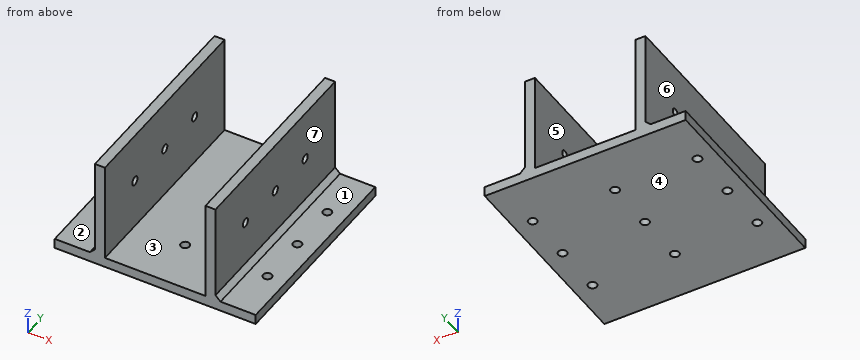
```python
from build123d import *

# Parameters (mm, degrees)
SKETCH1_W               = 100
SKETCH1_H               = 100
BOSS_EXTRUDE1_DEPTH     = 5
SKETCH2_W               = 5
SKETCH2_H               = 100
BOSS_EXTRUDE2_DEPTH     = 50
SKETCH3_R               = 2.15
CUT_EXTRUDE1_DEPTH      = 10
LPATTERN1_COUNT         = 3
LPATTERN1_PITCH         = 25
MIRROR2_COPY_1_SKETCH_R = 2.15
MIRROR2_COPY_1_DEPTH    = 10
MIRROR2_COPY_2_SKETCH_R = 2.15
MIRROR2_COPY_2_DEPTH    = 10
MIRROR3_COPY_1_SKETCH_R = 2.15
MIRROR3_COPY_1_DEPTH    = 10
MIRROR3_COPY_2_SKETCH_R = 2.15
MIRROR3_COPY_2_DEPTH    = 10
MIRROR3_COPY_3_SKETCH_R = 2.15
MIRROR3_COPY_3_DEPTH    = 10
MIRROR3_COPY_4_SKETCH_R = 2.15
MIRROR3_COPY_4_DEPTH    = 10
CHAMFER1_SIZE           = 2.5
SKETCH7_R               = 2.15
CUT_EXTRUDE2_DEPTH      = 60
SKETCH8_R               = 2.15
CUT_EXTRUDE3_DEPTH      = 60


with BuildPart() as part:
    # Sketch1 → Boss-Extrude1 (new body)
    with BuildSketch(Plane.XY):
        Rectangle(SKETCH1_W, SKETCH1_H)
    extrude(amount=BOSS_EXTRUDE1_DEPTH)

    # Sketch2 → Boss-Extrude2 (add)
    with BuildSketch(Plane.XY.offset(5)):
        with Locations((27.5, 0)):
            Rectangle(SKETCH2_W, SKETCH2_H)
    boss_extrude2 = extrude(amount=BOSS_EXTRUDE2_DEPTH)

    # Sketch3 → Cut-Extrude1 (cut)
    with BuildSketch(Plane(origin=(0, 0, 0), x_dir=(-1, 0, 0), z_dir=(0, 0, -1))):
        with Locations((0, 25)):
            Circle(SKETCH3_R)
    cut_extrude1 = extrude(amount=-CUT_EXTRUDE1_DEPTH, mode=Mode.SUBTRACT)

    # Mirror1: Boss-Extrude2 across plane
    add(boss_extrude2.mirror(Plane(origin=(0, 0, 0), x_dir=(0, 0, 1), z_dir=(1, 0, 0))))

    # LPattern1: Cut-Extrude1 ×3
    with Locations(*[(0, -i * LPATTERN1_PITCH, 0) for i in range(1, LPATTERN1_COUNT)]):
        add(cut_extrude1, mode=Mode.SUBTRACT)

    # Mirror2: Cut-Extrude1 across plane
    add(cut_extrude1.mirror(Plane(origin=(20.5, 0, 0), x_dir=(0, 0, 1), z_dir=(1, 0, 0))), mode=Mode.SUBTRACT)

    # Mirror2 copy 1 sketch → Mirror2 copy 1 (cut)
    with BuildSketch(Plane(origin=(41, -25, 0), x_dir=(1, 0, 0), z_dir=(0, 0, -1))):
        with Locations((0, -25)):
            Circle(MIRROR2_COPY_1_SKETCH_R)
    extrude(amount=-MIRROR2_COPY_1_DEPTH, mode=Mode.SUBTRACT)

    # Mirror2 copy 2 sketch → Mirror2 copy 2 (cut)
    with BuildSketch(Plane(origin=(41, -50, 0), x_dir=(1, 0, 0), z_dir=(0, 0, -1))):
        with Locations((0, -25)):
            Circle(MIRROR2_COPY_2_SKETCH_R)
    extrude(amount=-MIRROR2_COPY_2_DEPTH, mode=Mode.SUBTRACT)

    # Mirror3 copy 1 sketch → Mirror3 copy 1 (cut)
    with BuildSketch(Plane(origin=(-41, 0, 0), x_dir=(-1, 0, 0), z_dir=(0, 0, -1))):
        with Locations((0, 25)):
            Circle(MIRROR3_COPY_1_SKETCH_R)
    extrude(amount=-MIRROR3_COPY_1_DEPTH, mode=Mode.SUBTRACT)

    # Mirror3 copy 2 sketch → Mirror3 copy 2 (cut)
    with BuildSketch(Plane(origin=(-41, -25, 0), x_dir=(-1, 0, 0), z_dir=(0, 0, -1))):
        with Locations((0, 25)):
            Circle(MIRROR3_COPY_2_SKETCH_R)
    extrude(amount=-MIRROR3_COPY_2_DEPTH, mode=Mode.SUBTRACT)

    # Mirror3 copy 3 sketch → Mirror3 copy 3 (cut)
    with BuildSketch(Plane(origin=(-41, -50, 0), x_dir=(-1, 0, 0), z_dir=(0, 0, -1))):
        with Locations((0, 25)):
            Circle(MIRROR3_COPY_3_SKETCH_R)
    extrude(amount=-MIRROR3_COPY_3_DEPTH, mode=Mode.SUBTRACT)

    # Mirror3 copy 4 sketch → Mirror3 copy 4 (cut)
    with BuildSketch(Plane(origin=(0, 0, 0), x_dir=(1, 0, 0), z_dir=(0, 0, -1))):
        with Locations((0, -25)):
            Circle(MIRROR3_COPY_4_SKETCH_R)
    extrude(amount=-MIRROR3_COPY_4_DEPTH, mode=Mode.SUBTRACT)

    # Chamfer1
    chamfer1_edges = [part.edges().sort_by_distance(p)[0] for p in [
        (30, 0, 5),
        (-30, 0, 5),
    ]]
    chamfer(chamfer1_edges, length=CHAMFER1_SIZE)

    # Sketch7 → Cut-Extrude2 (cut)
    with BuildSketch(Plane.ZY.offset(30)):
        with Locations(Location((30, 25, 0), (0, 0, 270))):
            Circle(SKETCH7_R)
    cut_extrude2 = extrude(amount=-CUT_EXTRUDE2_DEPTH, mode=Mode.SUBTRACT)

    # Sketch8 → Cut-Extrude3 (cut)
    with BuildSketch(Plane.ZY.offset(30)):
        with Locations(Location((30, 0, 0), (0, 0, 270))):
            Circle(SKETCH8_R)
        with Locations(Location((30, 25, 0), (0, 0, 270))):
            Circle(SKETCH8_R)
    extrude(amount=-CUT_EXTRUDE3_DEPTH, mode=Mode.SUBTRACT)

    # Mirror4: Cut-Extrude2 across plane
    add(cut_extrude2.mirror(Plane.ZX), mode=Mode.SUBTRACT)


solid = part.part
```
Check sheet for the modelled part. Datum: model origin and axes. Units: mm. Face numbers are marked on the shaded views. A direction names the side the tool comes from. Coordinates: 2 decimals unless noted, no trailing zeros. Order: outer loops, then holes, each group sorted by start corner. A loop starts at its lowest first (then second) coordinate and runs counter-clockwise, first axis right, second up. Notation, with made-up numbers: (67, 21) -> (75, 21) arc R19 ccw to (75, 28) -> close; hole circle Ø5 at (17, -25). An arc over 180 degrees is marked (long way). Write each question's results on one line, items separated by ' | '. Start each with the question number.
1) Draft check along X on the marked faces 4, 5, 6 and 7. Enter one of: pulls with the +X half, pulls with the -X half, needs draft (parallel to the pull), parting line crosses it, or undercut.
2) Section check A-A (z = 30). Count the separate pieces of the cut face and the enclosed holes in it, and give its area (3 significant figures).
3) Depth check by flat-ended pin: pin 1 (3 mm diameter, centred on x = -7, y = -29, fed in from -Z); pin 2 (5 mm diameter, centred on y = 0, z = 30, fed in from +X); pin 3 (3.5 mm diameter, centred on x = -41, y = 25, fed in from -Z); pin 4 (8 mm diameter, centred on y = 7, z = 20, fed in from -X). Enter the tip coordinate at first touch or a pass-through.
4) Section check B-B (z = 43.5). Enter the section's corners in (x, y).
5) Set-up check for the marked faces 1, 2 and 3: record each of +Z, -Z, +X, -X, +Y, -Y from which the full face is reachable in a straight line by a thin tool's end or side.
6) Section check D-D (x = -41). Enter the section's corners in (y, z).
7) Material ranges on line 1 along Y through (x, z) = (41, 1); line 2 along X through (y, z) = (34.5, 50.5); line 3 along Z through (x, y) = (-28, 25), recorded low to high.
Checked values:
1) face 4: needs draft | face 5: undercut | face 6: pulls with the -X half | face 7: pulls with the +X half
2) separate pieces: 8 | enclosed holes: 0 | area: 871 mm²
3) pin 1: z = 0 | pin 2: x = 30 | pin 3: through | pin 4: x = -30
4) outline: (-30, -50) -> (-25, -50) -> (-25, 50) -> (-30, 50) -> close; (25, -50) -> (30, -50) -> (30, 50) -> (25, 50) -> close
5) face 1: +Z, +X, +Y, -Y | face 2: +Z, -X, +Y, -Y | face 3: +Z, +Y, -Y
6) outline: (-50, 0) -> (-27.15, 0) -> (-27.15, 5) -> (-50, 5) -> close; (-22.85, 0) -> (-2.15, 0) -> (-2.15, 5) -> (-22.85, 5) -> close; (2.15, 0) -> (22.85, 0) -> (22.85, 5) -> (2.15, 5) -> close; (27.15, 0) -> (50, 0) -> (50, 5) -> (27.15, 5) -> close
7) line 1: -50 to -27.15, -22.85 to -2.15, 2.15 to 22.85, 27.15 to 50 | line 2: -30 to -25, 25 to 30 | line 3: 0 to 27.85, 32.15 to 55
